Could you check a few things on this model? Use its own coordinates, in mm. A direction names the side the tool comes from. Coordinates: 2 decimals unless noted, no trailing zeros. Write each loop counter-clockwise with the first axis right and the second up, starting at its lowest first coordinate (ties: lowest second). Pieces come first, ordered by that corner, then holes. Notation, with made-up numbers: (-4, 0.5) - (14, 0.5) arc R5 cw to (14, 5.5) - close; hole circle Ø6 at (39.25, -13). An arc over 180 degrees is marked (long way). Answer as a JSON object with one key per item and string values. Group by question number.
1) On a 3-axis mill with a long thin cutter (end or side, diameter ignored), from which of +Z, -Z, +X, -X, +Y, -Y can I reach the whole of each face in a straight line? I mean faces 5 (the flat face through (89, 82.61, 2)), 6 (the cylindrical face through (93.925, 96.686, -15.675)), 7 (the flat face through (64, 55.841, -26)), 8 (the flat face through (78.92, 79, -26)). Say none if no direction works.
2) If we section it at C-C (x = 26.5): Write out the boundary of the cut face in (y, z).
3) If we section it at B-B (z = -50): Write out the boundary of the cut face in (x, y).
4) If we section it at A-A (y = 59.5): Write out the boundary of the cut face in (x, z), plus the area to 3 significant figures.
5) Please list where these lines run through material, in increasing order: line 1 along Z through (x, y) = (34.5, 43.5); line 2 along Z through (x, y) = (16, 76); line 3 along Z through (x, y) = (50, 33).
6) We'd pull the mould along Y, two halves only. Please class faces 1 (the flat face through (32, 33.46, 2)), 2 (the flat face through (49, 33.196, -77)), 3 (the flat face through (21.109, 78, 5)), 4 (the cylindrical face through (7.38, 24.02, 4.93)): released by +Y, released by -Y, zero draft, split by the parting line, or undercut.
7) Will these pins go through, and if not, where does the flat tip stop? pin 1 Ø1.5 at (x, y) = (64, 12.5) entering from -Z; pin 2 Ø4 at (x, z) = (69.5, -26.5) entering from +Y; pin 3 Ø10 at (x, y) = (33, 42) entering from +Z; pin 4 Ø0.9 at (y, z) = (62.5, 3.5) entering from +X.
```python
from build123d import *

# Parameters (mm, degrees)
CROQUIS1_W               = 100
CROQUIS1_H               = 100
SALIENTE_EXTRUIR1_DEPTH  = 100
CROQUIS2_W               = 25
CROQUIS2_H               = 100
CORTAR_EXTRUIR1_DEPTH    = 100
CROQUIS3_R               = 4
CORTAR_EXTRUIR2_DEPTH    = 100
CROQUIS4_R               = 2
SALIENTE_EXTRUIR2_DEPTH  = 100
CROQUIS5_W               = 28.014963793
CROQUIS5_H               = 9.051812895
CROQUIS5_W_2             = 2.954560647
CROQUIS5_W_3             = 3.39657131
CROQUIS5_W_4             = 2.705494987
CROQUIS5_W_5             = 11.571132933
CROQUIS5_H_2             = 11.097873227
SALIENTE_EXTRUIR3_DEPTH  = 5
CROQUIS6_R               = 3.840531475
CROQUIS6_R_2             = 4.686080108
SALIENTE_EXTRUIR4_DEPTH  = 15
CROQUIS7_W               = 38.87912129
CROQUIS7_H               = 26.349323358
SALIENTE_EXTRUIR5_DEPTH  = 15
CROQUIS9_R               = 4.785044561
CROQUIS9_R_2             = 6.367870478
CROQUIS9_R_3             = 2.466912166
SALIENTE_EXTRUIR7_DEPTH  = 10
CROQUIS10_R              = 5.793086174
CROQUIS10_R_2            = 2.31809738
CROQUIS10_R_3            = 5.48706726
CROQUIS10_R_4            = 3.763310936
CROQUIS10_W              = 32.541145419
CROQUIS10_H              = 7.810522345
CROQUIS10_W_2            = 51.521675343
CROQUIS10_H_2            = 23.571567841
SALIENTE_EXTRUIR8_DEPTH  = 10
CROQUIS11_R              = 6.618616789
CROQUIS11_R_2            = 4.139609283
CROQUIS11_R_3            = 2.844513546
CROQUIS11_W              = 11.477012866
CROQUIS11_H              = 22.393691404
CROQUIS11_W_2            = 15.030927027
CROQUIS11_H_2            = 13.868299131
SALIENTE_EXTRUIR9_DEPTH  = 10
CROQUIS12_W              = 8.359310308
CROQUIS12_H              = 1.309360747
CROQUIS12_H_2            = 1.067105011
CROQUIS12_H_3            = 1.50693684
CROQUIS12_H_4            = 1.336617059
SALIENTE_EXTRUIR12_DEPTH = 5
CROQUIS13_W              = 6.56197319
CROQUIS13_H              = 1.705437116
CROQUIS13_H_2            = 1.130487953
CROQUIS13_H_3            = 1.287425288
CROQUIS13_H_4            = 1.401382976
CROQUIS13_H_5            = 1.087508306
CROQUIS13_W_2            = 6.487517882
CROQUIS13_H_6            = 1.626101739
CROQUIS13_H_7            = 1.54333906
CROQUIS13_H_8            = 1.322914308
CROQUIS13_H_9            = 1.1734676
SALIENTE_EXTRUIR13_DEPTH = 5
CROQUIS14_W              = 30.712185141
CROQUIS14_H              = 20.943922245
CROQUIS14_W_2            = 19.421800597
CROQUIS14_H_2            = 1.175823789
CROQUIS14_W_3            = 20.78262229
CROQUIS14_H_3            = 1.282192639
CROQUIS14_W_4            = 20.500354159
CROQUIS14_H_4            = 0.874412394
CROQUIS14_W_5            = 18.507472387
CROQUIS14_H_5            = 1.583604033
CROQUIS14_W_6            = 21.149419091
CROQUIS14_H_6            = 1.323547308
SALIENTE_EXTRUIR14_DEPTH = 5


with BuildPart() as part:
    # Croquis1 → Saliente-Extruir1 (new body)
    with BuildSketch(Plane(origin=(0, 0, 0), x_dir=(1, 0, 0), z_dir=(0, 1, 0))):
        with Locations((50, 50)):
            Rectangle(CROQUIS1_W, CROQUIS1_H)
    extrude(amount=SALIENTE_EXTRUIR1_DEPTH)

    # Croquis2 → Cortar-Extruir1 (cut)
    with BuildSketch(Plane(origin=(100, 0, 0), x_dir=(0, 0, -1), z_dir=(1, 0, 0))):
        with Locations((15.5, 50)):
            Rectangle(CROQUIS2_W, CROQUIS2_H)
        with Locations((84.5, 50)):
            Rectangle(CROQUIS2_W, CROQUIS2_H)
    extrude(amount=-CORTAR_EXTRUIR1_DEPTH, mode=Mode.SUBTRACT)

    # Croquis3 → Cortar-Extruir2 (cut)
    with BuildSketch(Plane(origin=(0, 100, 0), x_dir=(1, 0, 0), z_dir=(0, 1, 0))):
        with Locations((50, 50)):
            Circle(CROQUIS3_R)
    extrude(amount=-CORTAR_EXTRUIR2_DEPTH, mode=Mode.SUBTRACT)

    # Croquis4 → Saliente-Extruir2 (add)
    with BuildSketch(Plane(origin=(0, 0, -100), x_dir=(-1, 0, 0), z_dir=(0, 0, -1))):
        with Locations((-95, 95)):
            Circle(CROQUIS4_R)
        with Locations((-95, 5.03405208)):
            Circle(CROQUIS4_R)
        with Locations((-5, 95)):
            Circle(CROQUIS4_R)
        with Locations((-5, 5.03405208)):
            Circle(CROQUIS4_R)
    extrude(amount=-SALIENTE_EXTRUIR2_DEPTH)

    # Croquis5 → Saliente-Extruir3 (add)
    with BuildSketch(Plane(origin=(0, 0, -100), x_dir=(-1, 0, 0), z_dir=(0, 0, -1))):
        with Locations((-23.635184558, 12.112124115)):
            Rectangle(CROQUIS5_W, CROQUIS5_H)
        with Locations((-52.541553902, 12.112124115)):
            Rectangle(CROQUIS5_W_2, CROQUIS5_H)
        with Locations((-59.50170842, 12.112124115)):
            Rectangle(CROQUIS5_W_3, CROQUIS5_H)
        with Locations((-73.987801173, 12.112124115)):
            Rectangle(CROQUIS5_W_4, CROQUIS5_H)
        with Locations((-58.32712037, 48.743140543)):
            Rectangle(CROQUIS5_W_5, CROQUIS5_H_2)
    extrude(amount=SALIENTE_EXTRUIR3_DEPTH)

    # Croquis6 → Saliente-Extruir4 (add)
    with BuildSketch(Plane(origin=(0, 0, -100), x_dir=(-1, 0, 0), z_dir=(0, 0, -1))):
        with Locations((-13.664728634, 30.653502261)):
            Circle(CROQUIS6_R)
        with Locations((-92.1488144, 26.812970786)):
            Circle(CROQUIS6_R_2)
    extrude(amount=SALIENTE_EXTRUIR4_DEPTH)

    # Croquis7 → Saliente-Extruir5 (add)
    with BuildSketch(Plane(origin=(0, 0, -100), x_dir=(-1, 0, 0), z_dir=(0, 0, -1))):
        with Locations((-25.561971547, 79.979772745)):
            Rectangle(CROQUIS7_W, CROQUIS7_H)
    extrude(amount=SALIENTE_EXTRUIR5_DEPTH)

    # Croquis9 → Saliente-Extruir7 (add)
    with BuildSketch(Plane(origin=(0, 0, -100), x_dir=(-1, 0, 0), z_dir=(0, 0, -1))):
        with Locations((-90.660928356, 84.874198192)):
            Circle(CROQUIS9_R)
        with Locations((-91.763562846, 71.404974806)):
            Circle(CROQUIS9_R_2)
        with Locations((-80.514248765, 84.874198192)):
            Circle(CROQUIS9_R_3)
    extrude(amount=SALIENTE_EXTRUIR7_DEPTH)

    # Croquis10 → Saliente-Extruir8 (add)
    with BuildSketch(Plane(origin=(0, 0, -72), x_dir=(-1, 0, 0), z_dir=(0, 0, -1))):
        with Locations((-82.051886177, 25.231528411)):
            Circle(CROQUIS10_R)
        with Locations((-14.982847097, 87.088662407)):
            Circle(CROQUIS10_R_2)
        with Locations((-30.0148444, 91.575948126)):
            Circle(CROQUIS10_R_3)
        with Locations((-92.648427406, 75.96536285)):
            Circle(CROQUIS10_R_4)
        with Locations((-46.28541711, 73.951827076)):
            Rectangle(CROQUIS10_W, CROQUIS10_H)
        with Locations((-49.06617746, 44.981737468)):
            Rectangle(CROQUIS10_W_2, CROQUIS10_H_2)
    extrude(amount=SALIENTE_EXTRUIR8_DEPTH)

    # Croquis11 → Saliente-Extruir9 (add)
    with BuildSketch(Plane.XY):
        with Locations((44.886334375, 89.290075512)):
            Circle(CROQUIS11_R)
        with Locations((10.869565611, 35.747288597)):
            Circle(CROQUIS11_R_2)
        with Locations((9.632332503, 25.754447062)):
            Circle(CROQUIS11_R_3)
        with Locations((15.370838936, 78.09322981)):
            Rectangle(CROQUIS11_W, CROQUIS11_H)
        with Locations((55.139514231, 55.011152001)):
            Rectangle(CROQUIS11_W_2, CROQUIS11_H_2)
    extrude(amount=SALIENTE_EXTRUIR9_DEPTH)

    # Croquis12 → Saliente-Extruir12 (add)
    with BuildSketch(Plane.XY):
        with Locations((32.266668911, 21.407969294)):
            Rectangle(CROQUIS12_W, CROQUIS12_H)
        with Locations((32.266668911, 24.947933784)):
            Rectangle(CROQUIS12_W, CROQUIS12_H_2)
        with Locations((32.266668911, 29.162648826)):
            Rectangle(CROQUIS12_W, CROQUIS12_H_3)
        with Locations((32.266668911, 34.127920992)):
            Rectangle(CROQUIS12_W, CROQUIS12_H_4)
    extrude(amount=SALIENTE_EXTRUIR12_DEPTH)

    # Croquis13 → Saliente-Extruir13 (add)
    with BuildSketch(Plane.XY):
        with Locations((88.754333095, 89.142527072)):
            Rectangle(CROQUIS13_W, CROQUIS13_H)
        with Locations((88.754333095, 84.881148844)):
            Rectangle(CROQUIS13_W, CROQUIS13_H_2)
        with Locations((88.754333095, 81.966755107)):
            Rectangle(CROQUIS13_W, CROQUIS13_H_3)
        with Locations((88.754333095, 78.33963479)):
            Rectangle(CROQUIS13_W, CROQUIS13_H_4)
        with Locations((88.754333095, 74.883451007)):
            Rectangle(CROQUIS13_W, CROQUIS13_H_5)
        with Locations((70.610389752, 74.070400138)):
            Rectangle(CROQUIS13_W_2, CROQUIS13_H_6)
        with Locations((70.610389752, 70.003046572)):
            Rectangle(CROQUIS13_W_2, CROQUIS13_H_7)
        with Locations((70.610389752, 66.51511908)):
            Rectangle(CROQUIS13_W_2, CROQUIS13_H_8)
        with Locations((70.610389752, 62.363953227)):
            Rectangle(CROQUIS13_W_2, CROQUIS13_H_9)
    extrude(amount=SALIENTE_EXTRUIR13_DEPTH)

    # Croquis14 → Saliente-Extruir14 (add)
    with BuildSketch(Plane.XY.offset(-28)):
        with Locations((63.563993269, 79.414556202)):
            Rectangle(CROQUIS14_W, CROQUIS14_H)
        with Locations((63.845595451, 56.428453676)):
            Rectangle(CROQUIS14_W_2, CROQUIS14_H_2)
        with Locations((64.526006297, 52.711211406)):
            Rectangle(CROQUIS14_W_3, CROQUIS14_H_3)
        with Locations((66.027962056, 48.736894588)):
            Rectangle(CROQUIS14_W_4, CROQUIS14_H_4)
        with Locations((67.024402941, 44.505503223)):
            Rectangle(CROQUIS14_W_5, CROQUIS14_H_5)
        with Locations((68.345376294, 40.563693497)):
            Rectangle(CROQUIS14_W_6, CROQUIS14_H_6)
    extrude(amount=SALIENTE_EXTRUIR14_DEPTH)


solid = part.part
```
Here are the results:
{
 "1": {"face 5": "+Z, +X", "face 6": "none", "face 7": "+X, -X", "face 8": "+X, +Y, -Y"},
 "2": {"outline": "(0, -100) - (7.59, -100) - (7.59, -105) - (16.64, -105) - (16.64, -100) - (66.81, -100) - (66.81, -115) - (93.15, -115) - (93.15, -100) - (100, -100) - (100, -97) - (0, -97) - close; (0, -72) - (33.2, -72) - (33.2, -82) - (56.77, -82) - (56.77, -72) - (87.36, -72) - (87.36, -82) - (95.79, -82) - (95.79, -72) - (100, -72) - (100, -28) - (0, -28) - close; (0, -3) - (100, -3) - (100, 0) - (0, 0) - close"},
 "3": {"outline": "(0, 0) - (46, 0) - (46, 100) - (0, 100) - close; (54, 0) - (100, 0) - (100, 100) - (54, 100) - close"},
 "4": {"outline": "(0, -100) - (100, -100) - (100, -97) - (0, -97) - close; (0, -72) - (100, -72) - (100, -28) - (0, -28) - close; (0, -3) - (100, -3) - (100, 0) - (62.65, 0) - (62.65, 10) - (47.62, 10) - (47.62, 0) - (0, 0) - close; hole circle Ø8 at (50, -50)", "area": "5,100 mm²"},
 "5": {"line 1": "z = -100 to -97, -82 to -28, -3 to 0", "line 2": "z = -115 to -97, -72 to -28, -3 to 10", "line 3": "z = -100 to -97, -72 to -54, -46 to -28, -3 to 0"},
 "6": {"face 1": "undercut", "face 2": "released by -Y", "face 3": "zero draft", "face 4": "undercut"},
 "7": {"pin 1": "stops at z = -100", "pin 2": "stops at y = 100", "pin 3": "stops at z = 0", "pin 4": "stops at x = 73.85"}
}
